```python
from build123d import *

# Parameters (mm, degrees)
F0_R     = 4.5
F0_W     = 12
F0_H     = 3
F1_DEPTH = 2
F2_R     = 5.5
F3_DEPTH = 0.5
F5_R     = 1.49999
F7_DEPTH = 25
F8_R     = 3


# Not quite as in the source:
# - a fillet or chamfer is up to 0.001 mm smaller than in the source, because OpenCascade refuses the exact size


with BuildPart() as f1:
    # F0 (on Top) → F1 (new body)
    with BuildSketch(Plane.XY):
        Polygon((14.4337567297, -25), (28.8675134595, 0), (14.4337567297, 25), (-14.4337567297, 25), (-28.8675134595, 0), (-14.4337567297, -25), align=None)
        with Locations((9.37942788, 7.2647714987)):
            Circle(F0_R, mode=Mode.SUBTRACT)
        with Locations((0.0337567297, 21)):
            Rectangle(F0_W, F0_H, mode=Mode.SUBTRACT)
    extrude(amount=F1_DEPTH)

    # F2 (on face) → F3 (cut)
    with BuildSketch(Plane.XY.offset(2)):
        Polygon((-13.8564064606, -24), (13.8564064606, -24), (27.7128129211, 0), (17.0318329411, 18.5), (-17.0318329411, 18.5), (-27.7128129211, 0), align=None)
        with Locations((9.37942788, 7.2647714987)):
            Circle(F2_R, mode=Mode.SUBTRACT)
    extrude(amount=-F3_DEPTH, mode=Mode.SUBTRACT)

    # F5 (radius 1.5 in the source; OpenCascade refuses exactly that, so slightly less here)
    f5_edges = [f1.edges().sort_by_distance(p)[0] for p in [
        (-5.966243, 19.5, 1),
        (6.033757, 19.5, 1),
        (6.033757, 22.5, 1),
        (-5.966243, 22.5, 1),
        (-17.031833, 18.5, 1.75),
        (-27.712813, 0, 1.75),
        (17.031833, 18.5, 1.75),
        (27.712813, 0, 1.75),
    ]]
    fillet(f5_edges, radius=F5_R)

    # F6 (on face) → F7 (cut)
    with BuildSketch(Plane.XY.offset(2)):
        with BuildLine():
            Line((-4.4662432703, 25.5), (4.5337567297, 25.5))
            ThreePointArc((4.5337567297, 25.5), (7.5909047219, 24.3020972357), (9.0204233671, 21.3461538462))
            ThreePointArc((9.0204233671, 21.3461538462), (9.6557649872, 20.0324012286), (11.0144974281, 19.5))
            Line((11.0144974281, 19.5), (21.36195996, 19.5))
            Line((21.36195996, 19.5), (25.703800239, 29.2692627907))
            Line((25.703800239, 29.2692627907), (-20.3538952839, 30.2788760662))
            Line((-20.3538952839, 30.2788760662), (-17.6091832103, 19.5))
            Line((-17.6091832103, 19.5), (-10.9469839687, 19.5))
            ThreePointArc((-10.9469839687, 19.5), (-9.5882515277, 20.0324012286), (-8.9529099076, 21.3461538462))
            ThreePointArc((-8.9529099076, 21.3461538462), (-7.5233912624, 24.3020972357), (-4.4662432703, 25.5))
        make_face()
    extrude(amount=-F7_DEPTH, mode=Mode.SUBTRACT)

    # F8
    f8_edges = [f1.edges().sort_by_distance(p)[0] for p in [
        (-6.527796, 25, 1),
        (6.59531, 25, 1),
    ]]
    fillet(f8_edges, radius=F8_R)


solid = f1.part
```
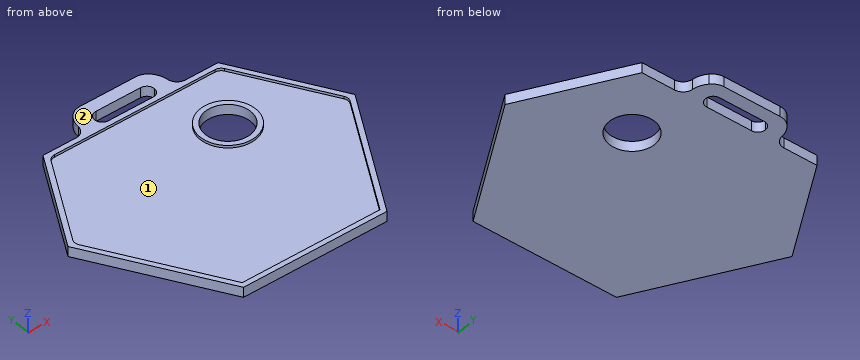
Check sheet for the modelled part. Datum: model origin and axes. Units: mm. Face numbers are marked on the shaded views. Coordinates: 2 decimals unless noted, no trailing zeros. Loops run counter-clockwise (first coordinate to the right, second up) from the corner with the lowest first, then second, coordinate; pieces in that order, holes last.
1) Material ranges on probe 1 along Y at (x, z) = (2, 1.4); probe 2 along X at (y, z) = (4, 1.75); probe 3 along Y at (x, z) = (8, 1.75), recorded low to high.
2) Gauge pin test, flat ends, axial feed: pin 1 (0.6 mm diameter, centred on x = -15.5, z = 0.5, fed in from +Y); pin 2 (1.5 mm diameter, centred on x = -18, y = 7.5, fed in from +Z). Record the tip position at first contact, or that the pin passes through.
3) Release check for a two-part mould opening along X. For the marked faces 1 and 2 record: released by +X, released by -X, zero draft, split by the parting line, or undercut.
4) Sectioned sample at B-B (x = -13). Record the boundary of the cut face in (y, z), and give its area (4 significant figures).
5) Sectioned sample at A-A (z = 0.4). Count the separate pieces of the cut face and the enclosed holes in it, and give its area (3 significant figures).
6) Sectioned sample at C-C (y = 15.5). Record the boundary of the cut face in (x, z), and give its area (3 significant figures).
Check sheet entries:
1. probe 1: y = -25 to 19.5, 22.5 to 25
1. probe 2: x = -26.56 to -25.4, 4.95 to 6.28, 12.48 to 13.81, 25.4 to 26.56
1. probe 3: y = -25 to -24, 1.94 to 2.98, 11.55 to 12.59, 18.5 to 23.87
2. pin 1: stops at y = 19.5
2. pin 2: stops at z = 1.5
3. face 1: undercut
3. face 2: zero draft
4. outline: (-25, 0) - (19.5, 0) - (19.5, 2) - (18.5, 2) - (18.5, 1.5) - (-24, 1.5) - (-24, 2) - (-25, 2) - close
4. area: 67.75 mm2
5. separate pieces: 1
5. enclosed holes: 2
5. area: 1,990 mm2
6. outline: (-19.92, 0) - (19.92, 0) - (19.92, 2) - (18.76, 2) - (18.76, 1.5) - (-18.76, 1.5) - (-18.76, 2) - (-19.92, 2) - close
6. area: 60.9 mm2
